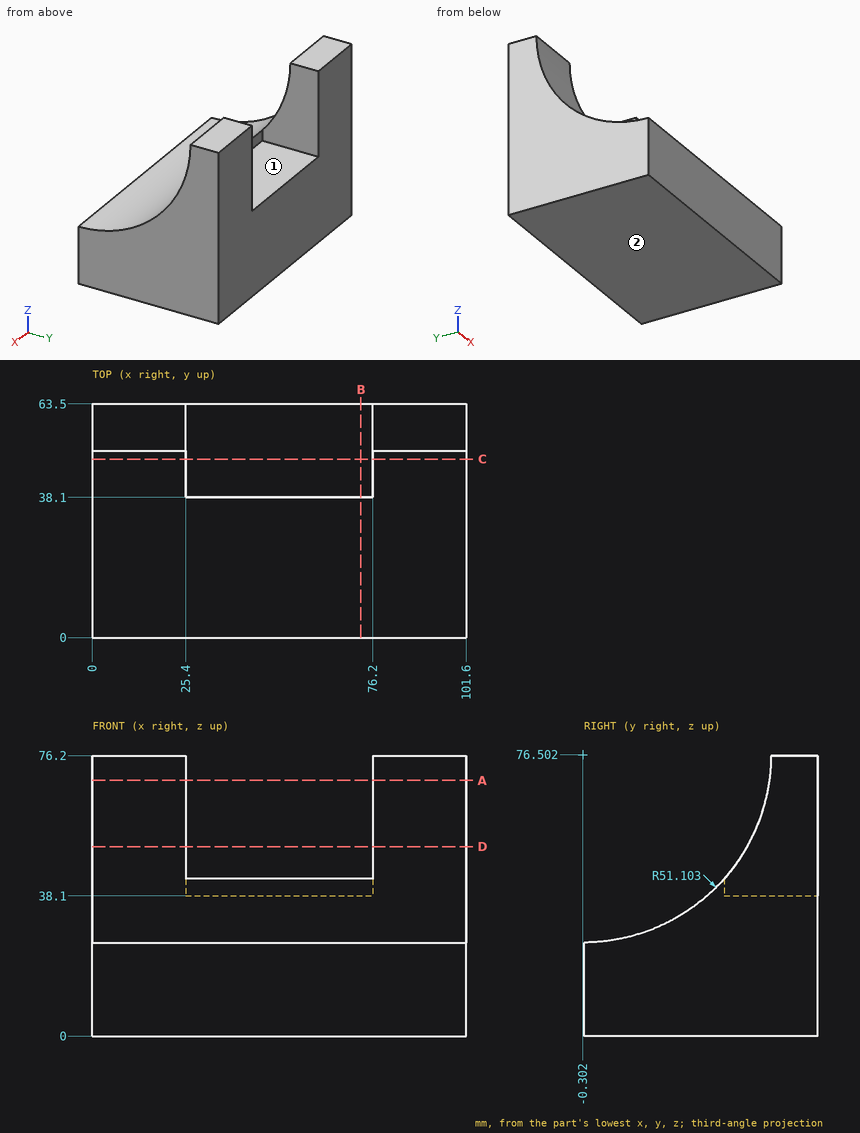
For this review, use the dimensioned drawing (mm, ordinates from the lowest corner) and the shaded views. A direction names the side the tool comes from. Round coordinates to 2 decimals unless told otherwise and drop trailing zeros. Order: outer loops, then holes, each group sorted by start corner. A loop starts at its lowest first (then second) coordinate and runs counter-clockwise, first axis right, second up. Notation, with made-up numbers: (26, 24.25) -> (76, 24.25) arc R31 cw to (76, 52.25) -> close; hole circle Ø8 at (36, -27.75). An arc over 180 degrees is marked (long way). One line per item, written item: value. Start each with the question number.
Q1. Take a section at A-A (z = 69.5). Write out the cut boundary in (x, y), and give its area (3 significant figures).
Q2. Take a section at C-C (y = 48.5). Write out the cut boundary in (x, z).
Q3. Clearance check with flat-ended pins moving along their axes: pin 1 Ø2.5 at (x, z) = (47.5, 41) entering from +Y; pin 2 Ø1 at (x, z) = (10.5, 45.5) entering from -Y; pin 3 Ø6 at (x, y) = (55, 41) entering from +Z; pin 4 Ø5 at (x, y) = (74, 52.5) entering from -Z. State where each tip first meets the part, or that it passes through.
Q4. Take a section at B-B (x = 73). Write out the cut boundary in (y, z).
Q5. Wall thickness on line 1 (Z direction, x = 51, y = 58.5); line 2 (Z direction, x = 43.5, y = 20) (3 decimals); line 3 (Y direction, x = 44.5, z = 35) (1 decimal): over which ranges is each line inside the solid? List them lowest first.
Q6. Machinability: for the marked faces 1 and 2, which of the approach directions +Z, -Z, +X, -X, +Y, -Y give a long, thin tool a straight path to every point of the face, cutting with its end or side? Answer none if there is none.
Q7. Take a section at D-D (z = 51.5). Write out the cut boundary in (x, y).
Reported:
1. outline: (0, 50.32) -> (25.4, 50.32) -> (25.4, 63.5) -> (0, 63.5) -> close; (76.2, 50.32) -> (101.6, 50.32) -> (101.6, 63.5) -> (76.2, 63.5) -> close
1. area: 670 mm2
2. outline: (0, 0) -> (101.6, 0) -> (101.6, 61.34) -> (76.2, 61.34) -> (76.2, 38.1) -> (25.4, 38.1) -> (25.4, 61.34) -> (0, 61.34) -> close
3. pin 1: stops at y = 38.1
3. pin 2: stops at y = 39.94
3. pin 3: stops at z = 42.79
3. pin 4: stops at z = 0
4. outline: (0, 0) -> (63.5, 0) -> (63.5, 38.1) -> (38.1, 38.1) -> (38.1, 42.79) arc R51.1 cw to (0, 25.4) -> close
5. line 1: z = 0 to 38.1
5. line 2: z = 0 to 29.605
5. line 3: y = 29.5 to 63.5
6. face 1: +Z, +Y
6. face 2: -Z, +X, -X, +Y, -Y
7. outline: (0, 44.27) -> (25.4, 44.27) -> (25.4, 63.5) -> (0, 63.5) -> close; (76.2, 44.27) -> (101.6, 44.27) -> (101.6, 63.5) -> (76.2, 63.5) -> close
